```python
from build123d import *


with BuildPart() as f1:
    # F0 (on Front) → F1 (revolve)
    with BuildSketch(Plane.XZ):
        with BuildLine():
            Line((0, -16.904561), (0, -12.7))
            ThreePointArc((0, -12.7), (-1.65751, -12.591372), (-3.286666, -12.267348))
            Line((-3.286666, -12.267348), (0, -16.904561))
        make_face()
        with BuildLine():
            Line((-7.27579, -15.094675), (-3.286666, -12.267348))
            ThreePointArc((-3.286666, -12.267348), (-5.362321, -11.512407), (-7.27579, -10.409269))
            Line((-7.27579, -10.409269), (-7.27579, -15.094675))
        make_face()
        with BuildLine():
            Line((-12.250861, -11.988905), (-7.27579, -10.409269))
            ThreePointArc((-7.27579, -10.409269), (-9.268421, -8.682533), (-10.861549, -6.581547))
            Line((-10.861549, -6.581547), (-12.250861, -11.988905))
        make_face()
        with BuildLine():
            Line((0, 0), (0, 12.7))
            ThreePointArc((0, 12.7), (-2.020944, 12.538173), (-3.990386, 12.056816))
            ThreePointArc((-3.990386, 12.056816), (-6.204223, 11.081409), (-8.192936, 9.703906))
            ThreePointArc((-8.192936, 9.703906), (-9.940865, 7.903746), (-11.30076, 5.795069))
            ThreePointArc((-11.30076, 5.795069), (-12.692011, -0.450404), (-10.861549, -6.581547))
            ThreePointArc((-10.861549, -6.581547), (-9.268421, -8.682533), (-7.27579, -10.409269))
            ThreePointArc((-7.27579, -10.409269), (-5.362321, -11.512407), (-3.286666, -12.267348))
            ThreePointArc((-3.286666, -12.267348), (-1.65751, -12.591372), (0, -12.7))
            Line((0, -12.7), (0, 0))
        make_face()
        with BuildLine():
            ThreePointArc((-10.861549, -6.581547), (-12.692011, -0.450404), (-11.30076, 5.795069))
            Line((-11.30076, 5.795069), (-14.924208, 5.795069))
            Line((-14.924208, 5.795069), (-13.112484, 0))
            Line((-13.112484, 0), (-14.559376, -5.631464))
            Line((-14.559376, -5.631464), (-10.861549, -6.581547))
        make_face()
        with BuildLine():
            ThreePointArc((-11.30076, 5.795069), (-9.940865, 7.903746), (-8.192936, 9.703906))
            Line((-8.192936, 9.703906), (-12.747521, 12.056816))
            Line((-12.747521, 12.056816), (-11.30076, 5.795069))
        make_face()
        with BuildLine():
            ThreePointArc((-8.192936, 9.703906), (-6.204223, 11.081409), (-3.990386, 12.056816))
            Line((-3.990386, 12.056816), (-8.192936, 15.187172))
            Line((-8.192936, 15.187172), (-8.192936, 9.703906))
        make_face()
        with BuildLine():
            ThreePointArc((-3.990386, 12.056816), (-2.020944, 12.538173), (0, 12.7))
            Line((0, 12.7), (-3.990386, 18.317528))
            Line((-3.990386, 18.317528), (-3.990386, 12.056816))
        make_face()
    revolve(axis=Axis((0, 0, -6.35), (0, 0, -1)))


solid = f1.part
```
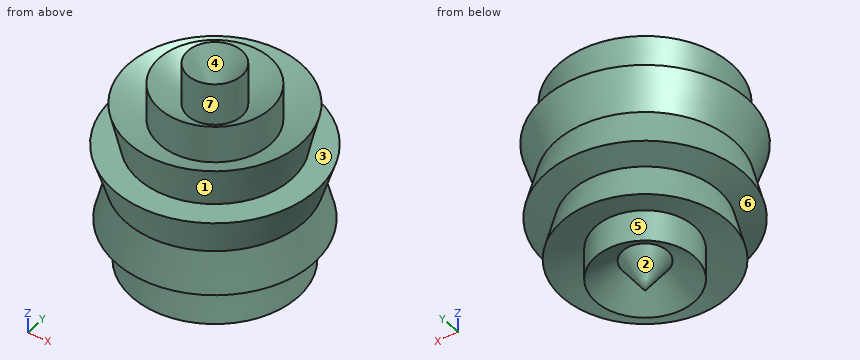
Geometry: final body of the model. Coordinates: model frame, mm. Face numbers are marked on the shaded views. A direction names the side the tool comes from. Round coordinates to 2 decimals unless told otherwise and drop trailing zeros. Loops run counter-clockwise (first coordinate to the right, second up) from the corner with the lowest first, then second, coordinate; pieces in that order, holes last. Notation, with made-up numbers: (34, -37.5) -> (83, -37.5) arc R17 ccw to (83, -14.5) -> close; hole circle Ø5 at (60.25, -26.75). An arc over 180 degrees is marked (long way). Use one line per item in the form item = value.
Item 1: Cut plane B-B on z = 16. Output: boundary loops of the cut face in (x, y).
Evaluation:
outline = circle Ø7.98 at (0, 0); hole circle Ø4.69 at (0, 0)
Item 2: Contact query for flat-ended pins moving along their axis: pin 1 Ø5 at (y, z) = (3.5, 0) entering from +X; pin 2 Ø5 at (x, z) = (-11, 2) entering from +Y; pin 3 Ø1 at (y, z) = (-6, -4) entering from +X. Output: stop coordinate, or through.
Evaluation:
pin_1 = 13.61
pin_2 = 11.03
pin_3 = 13.07
Item 3: Cut plane A-A on y = 11.5. Give the number of separate pieces and of enclosed holes in the cut face, then the cut area to 3 significant figures.
Evaluation:
separate_pieces = 3
enclosed_holes = 0
area = 238 mm2
Item 4: Draft query along Y for the marked faces 1, 2, 3 and 4. Return one class per face: released by +Y, released by -Y, zero draft, split by the parting line, or undercut.
Evaluation:
face_1 = split by the parting line
face_2 = undercut
face_3 = zero draft
face_4 = undercut
Item 5: Material intervals for probe 1 along Y at (x, z) = (4.5, 15); probe 2 along Z at (x, y) = (2, 3); probe 3 along Y at (x, z) = (-6.5, 2), sorted ascending.
Evaluation:
probe_1 = -6.85 to -6.54, 6.54 to 6.85
probe_2 = -12.49 to 17.78
probe_3 = -12.1 to 12.1
Item 6: Access query for the marked faces 5, 6 and 7. Directions: +Z, -Z, +X, -X, +Y, -Y. A direction counts if a zero-diameter tool reaches every point of the face in a straight line with its end or side. Return the directions, or none.
Evaluation:
face_5 = -Z
face_6 = none
face_7 = +Z
